Geometry check sheet. Reference: the model listing, model coordinates, mm. Face numbers are marked on the shaded views. Round coordinates to 2 decimals unless told otherwise and drop trailing zeros. Order: outer loops, then holes, each group sorted by start corner. A loop starts at its lowest first (then second) coordinate and runs counter-clockwise, first axis right, second up.
(1) Sectioned sample at B-B (z = 0). Record the boundary of the cut face in (x, y).
(2) Release check for a two-part mould opening along X. For the marked faces 1 and 2 record: +X half, -X half, draft (parallel to the pull), parting line (faces both ways), or undercut.
(3) Go/stop test with flat-tipped pins: pin 1 (2 mm diameter, centred on y = 3.5, z = -50.5, fed in from +X); pin 2 (2 mm diameter, centred on y = 7.5, z = -33, fed in from -X); pin 3 (1.5 mm diameter, centred on y = -0.5, z = -12, fed in from +X); pin 4 (11.5 mm diameter, centred on x = -2, z = -26, fed in from -Y). Record where each tip stops, or that it passes through.
(4) Sectioned sample at C-C (z = -54.5). Record the boundary of the cut face in (x, y).
(5) Sectioned sample at A-A (x = -7.5). Record the boundary of the cut face in (y, z).
(6) Material ranges on line 1 along Y through (x, z) = (-1, -7.5); line 2 along X through (y, z) = (1.25, -2); line 3 along X through (y, z) = (6, -78.5), recorded low to high.
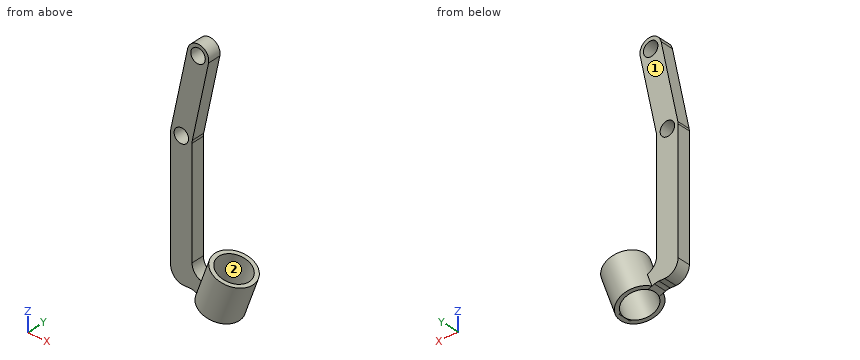
from build123d import *

# Parameters (mm, degrees)
SKETCH1_R           = 2.7
BOSS_EXTRUDE2_DEPTH = 5
FILLET2_R           = 5
SKETCH2_R           = 7.5
SKETCH2_R_2         = 6
BOSS_EXTRUDE3_DEPTH = 15
CUT_EXTRUDE1_DEPTH  = 15


with BuildPart() as part:
    # Sketch1 → Boss-Extrude2 (new body)
    with BuildSketch(Plane(origin=(0, 0, 0), x_dir=(1, 0, 0), z_dir=(0, 1, 0))):
        with BuildLine():
            Line((-10.149941127, 28.512781259), (-3.912590403, -0.831646763))
            ThreePointArc((-3.912590403, -0.831646763), (0.831646763, -3.912590403), (3.912590403, 0.831646763))
            Line((3.912590403, 0.831646763), (-2.237350725, 29.764844963))
            Line((-2.237350725, 29.764844963), (-2.237350725, 74.02353916))
            Line((-2.237350725, 74.02353916), (13.568139304, 79.776267068))
            Line((13.568139304, 79.776267068), (11.858038587, 84.474730172))
            Line((11.858038587, 84.474730172), (-2.237350725, 79.344428022))
            Line((-2.237350725, 79.344428022), (-10.237350725, 79.344428022))
            Line((-10.237350725, 79.344428022), (-10.237350725, 29.344428022))
            ThreePointArc((-10.237350725, 29.344428022), (-10.215438306, 28.926314169), (-10.149941127, 28.512781259))
        make_face()
        with Locations((-6.237350725, 29.344428022)):
            Circle(SKETCH1_R, mode=Mode.SUBTRACT)
        Circle(SKETCH1_R, mode=Mode.SUBTRACT)
    extrude(amount=BOSS_EXTRUDE2_DEPTH)

    # Fillet2
    fillet2_edges = [part.edges().sort_by_distance(p)[0] for p in [
        (-2.237350725, 2.5, -29.764844963),
        (-10.237350725, 2.5, -79.344428022),
        (-2.237350725, 2.5, -79.344428022),
        (-2.237350725, 2.5, -74.02353916),
    ]]
    fillet(fillet2_edges, radius=FILLET2_R)

    # Sketch2 → Boss-Extrude3 (add)
    with BuildSketch(Plane(origin=(-25.762527932, 0, -70.781963762), x_dir=(-0.939692621, 0, 0.342020143), z_dir=(-0.342020143, 0, -0.939692621))):
        with Locations((-34.010040431, 2.5)):
            Circle(SKETCH2_R)
        with Locations((-34.010040431, 2.5)):
            Circle(SKETCH2_R_2, mode=Mode.SUBTRACT)
    extrude(amount=-BOSS_EXTRUDE3_DEPTH)

    # Sketch2_2 → Cut-Extrude1 (cut)
    with BuildSketch(Plane(origin=(-25.762527932, 0, -70.781963762), x_dir=(-0.939692621, 0, 0.342020143), z_dir=(-0.342020143, 0, -0.939692621))):
        with BuildLine():
            ThreePointArc((-28.010040431, 2.5), (-28.148038369, 3.779426367), (-28.555684374, 5))
            Line((-28.555684374, 5), (-39.464396489, 5))
            ThreePointArc((-39.464396489, 5), (-40.010040431, 2.5), (-39.464396489, 0))
            Line((-39.464396489, 0), (-28.555684374, 0))
            ThreePointArc((-28.555684374, 0), (-28.148038369, 1.220573633), (-28.010040431, 2.5))
        make_face()
    extrude(amount=-CUT_EXTRUDE1_DEPTH, mode=Mode.SUBTRACT)


solid = part.part
Answer below:
1. outline: (-4.09, 0) - (-2.7, 0) - (-2.7, 5) - (-4.09, 5) - close; (2.7, 0) - (4, 0) - (4, 5) - (2.7, 5) - close
2. face 1: draft
2. face 2: undercut
3. pin 1: stops at x = -2.24
3. pin 2: passes through
3. pin 3: stops at x = 1.66
3. pin 4: stops at y = 0
4. outline: (-10.24, 0) - (-2.24, 0) - (-2.24, 5) - (-10.24, 5) - close
5. outline: (0, -78.8) - (5, -78.8) - (5, -31.73) - (0, -31.73) - close; (0, -26.96) - (5, -26.96) - (5, -16.05) - (0, -16.05) - close
6. line 1: y = 0 to 5
6. line 2: x = -4.51 to -1.81, 1.81 to 3.66
6. line 3: x = 0.56 to 2.43, 12.81 to 14.68
